Here's how the part is built. I have some questions about the finished solid (model axes, mm). A direction names the side the tool comes from. Give positions to 0.01 mm unless a question says otherwise; leave off trailing zeros. Write each loop counter-clockwise with the first axis right and the second up, starting at its lowest first coordinate (ties: lowest second). Pieces come first, ordered by that corner, then holes. Notation, with made-up numbers: M 5.5,73.25 L 23.5,73.25 A23 ccw 23.5,83.25 Z; hole C 60.5,73.25 d4. An arc over 180 degrees is marked long. Answer as CSV lines item,"result". Start each with the question number.
Q1. Thinking about a two-plate mould opening in Y: for faces 1 (the cylindrical face through (0, -30, 20)), 2 (the cylindrical face through (7.149, -43.044, 23.749)), 3 (the cylindrical face through (35, -10, 2)), 4 (the cylindrical face through (50, -10, 2)), which applies, +Y half, -Y half, draft (parallel to the pull), parting line (faces both ways), or undercut?
Q2. Suppose I cut it at C-C (x = 41). Write out the boundary of the cut face in (y, z).
Q3. On a 3-axis mill with a long thin cutter (end or side, diameter ignored), from which of +Z, -Z, +X, -X, +Y, -Y can I reach the whole of each face in a straight line? I mean faces 5 (the flat face through (35, -8, 5)), 6 (the flat face through (-20, -60, 14)), 7 (the cylindrical face through (-6.993, -42.889, 23.749)), 8 (the flat face through (-35, -12, 5)), 9 (the flat face through (1, 0, 21)). Say none if no direction works.
Q4. Suppose I cut it at B-B (z = 15). Write out the boundary of the cut face in (x, y).
Q5. Suppose I cut it at A-A (y = -10). Write out the boundary of the cut face in (x, z), then the cut area to 3 significant figures.
Q6. Suppose I cut it at D-D (y = -35). Write out the boundary of the cut face in (x, z), then the cut area to 3 significant figures.
Q7. If I drill on line 1 along X through (y, z) = (-10, 2.4); line 2 along Y through (x, z) = (-40, 3.4); line 3 along X through (y, z) = (-10, 1.05), over which ranges is the centre line in solid material (lowest first)?
Q8. For pin 1 (3 mm diameter, centred on y = -56.5, z = 22, fed in from -X); pin 2 (12 mm diameter, centred on x = 10, y = -8, fed in from +Z); pin 3 (4 mm diameter, centred on x = -26.5, z = 5, fed in from +Y); pin 4 (6 mm diameter, centred on y = -52.5, z = 12.5, fed in from -X), each with a flat end and sliding along its axis, tell me the tip position at first contact or that it passes through.
```python
from build123d import *

# Parameters (mm, degrees)
F1_DEPTH  = 60
F3_DEPTH  = 5
F4_R      = 5
F5_DEPTH  = 30.001
F6_W      = 20
F6_H      = 20
F7_DEPTH  = 30.001
F8_R      = 9.999
F10_DEPTH = 60.0010001


# Not quite as in the source:
# - a fillet or chamfer is up to 0.001 mm smaller than in the source, because OpenCascade refuses the exact size


with BuildPart() as f1:
    # F0 (on Front) → F1 (new body)
    with BuildSketch(Plane.XZ):
        with BuildLine():
            Line((-30, 0), (30, 0))
            ThreePointArc((30, 0), (0, 30), (-30, 0))
        make_face()
    extrude(amount=F1_DEPTH)

    # F2 (on Top) → F3 (join)
    with BuildSketch(Plane.XY):
        with BuildLine():
            Line((40, 0), (-40, 0))
            ThreePointArc((-40, 0), (-50, -10), (-40, -20))
            Line((-40, -20), (40, -20))
            ThreePointArc((40, -20), (50, -10), (40, 0))
        make_face()
    extrude(amount=F3_DEPTH)

    # F4 (on Top) → F5 (cut, through all)
    with BuildSketch(Plane.XY):
        with Locations((-40, -10)):
            Circle(F4_R)
        with Locations((40, -10)):
            Circle(F4_R)
    extrude(amount=F5_DEPTH, mode=Mode.SUBTRACT)

    # F6 (on Top) → F7 (cut, through all)
    with BuildSketch(Plane.XY):
        with Locations((0, -50.0372105837)):
            Rectangle(F6_W, F6_H)
    extrude(amount=F7_DEPTH, mode=Mode.SUBTRACT)

    # F8 (radius 10 in the source; OpenCascade refuses exactly that, so slightly less here)
    f8_edges = [f1.edges().sort_by_distance(p)[0] for p in [
        (-10, -40.037211, 14.142136),
        (10, -40.037211, 14.142136),
    ]]
    fillet(f8_edges, radius=F8_R)

    # F9 (on face) → F10 (cut, through all)
    with BuildSketch(Plane(origin=(0, 0, 0), x_dir=(-1, 0, 0), z_dir=(0, 1, 0))):
        with BuildLine():
            Line((-20, 0), (20, 0))
            ThreePointArc((20, 0), (0, 20), (-20, 0))
        make_face()
    extrude(amount=-F10_DEPTH, mode=Mode.SUBTRACT)


solid = f1.part
```
Resolved:
1,face 1,"draft"
1,face 2,"-Y half"
1,face 3,"undercut"
1,face 4,"parting line"
2,outline,"M -19.95,0 L -14.9,0 L -14.9,5 L -19.95,5 Z; M -5.1,0 L -0.05,0 L -0.05,5 L -5.1,5 Z"
3,face 5,"+Z, +X, +Y, -Y"
3,face 6,"+Z, -Z, +X, -X, -Y"
3,face 7,"+Z, -Z, -Y"
3,face 8,"+Z, -X, +Y, -Y"
3,face 9,"+Z, -Z, +X, -X, +Y"
4,outline,"M -25.98,-60 L -13.23,-60 L -13.23,0 L -25.98,0 Z; M 13.23,-60 L 25.98,-60 L 25.98,0 L 13.23,0 Z"
5,outline,"M -50,0 L -45,0 L -45,5 L -50,5 Z; M -35,0 L -20,0 A20 cw 20,0 L 35,0 L 35,5 L 29.58,5 A30 ccw -29.58,5 L -35,5 Z; M 45,0 L 50,0 L 50,5 L 45,5 Z"
5,area,"887 mm^2"
6,outline,"M -30,0 L -20,0 A20 cw 20,0 L 30,0 A30 ccw Z"
6,area,"785 mm^2"
7,line 1,"-50 to -45, -35 to -19.86, 19.86 to 35, 45 to 50"
7,line 2,"-20 to -15, -5 to 0"
7,line 3,"-50 to -45, -35 to -19.97, 19.97 to 35, 45 to 50"
8,pin 1,"x = -21.9"
8,pin 2,"z = 29.73"
8,pin 3,"y = 0"
8,pin 4,"x = -28.46"
